Geometry check sheet. Reference: the model listing, model coordinates, mm. Give positions to 0.01 mm unless a question says otherwise; leave off trailing zeros. Loops run counter-clockwise (first coordinate to the right, second up) from the corner with the lowest first, then second, coordinate; pieces in that order, holes last. Notation, with made-up numbers: (-29, 39.25) -> (-2, 39.25) arc R10 ccw to (-2, 45.25) -> close; hole circle Ø11 at (89, -2.5). An arc over 180 degrees is marked (long way). One line per question, with ' | ' between items.
from build123d import *

# Parameters (mm, degrees)
F0_R     = 10
F0_R_2   = 1.75
F1_DEPTH = 3
F2_SIZE  = 0.5
F3_SIZE2 = 0.6
F3_SIZE  = 0.4


with BuildPart() as f1:
    # F0 (on Right) → F1 (new body)
    with BuildSketch(Plane.YZ):
        Circle(F0_R)
        with Locations((0, -6.35)):
            Circle(F0_R_2, mode=Mode.SUBTRACT)
        with Locations((-6.35, 0)):
            Circle(F0_R_2, mode=Mode.SUBTRACT)
        with Locations((6.35, 0)):
            Circle(F0_R_2, mode=Mode.SUBTRACT)
        with Locations((0, 6.35)):
            Circle(F0_R_2, mode=Mode.SUBTRACT)
    extrude(amount=F1_DEPTH)

    # F2
    f2_edges = [f1.edges().sort_by_distance(p)[0] for p in [
        (3, -8.1, 0),
        (3, -1.75, 6.35),
        (3, 4.6, 0),
        (3, -1.75, -6.35),
    ]]
    chamfer(f2_edges, length=F2_SIZE)

    # F3
    f3_edges = [f1.edges().sort_by_distance(p)[0] for p in [
        (3, -10, 0),
        (0, -10, 0),
    ]]
    chamfer(f3_edges, length=F3_SIZE, length2=F3_SIZE2)


solid = f1.part
Item 1: Scan lines: probe 1 along Z at (x, y) = (2.05, 0); probe 2 along Y at (x, z) = (1.45, 0.5); probe 3 along Z at (x, y) = (2.7, -6). Record each from-to range of solid material in increasing order.
Result:
probe 1: -10 to -8.1, -4.6 to 4.6, 8.1 to 10 | probe 2: -9.99 to -8.03, -4.67 to 4.67, 8.03 to 9.99 | probe 3: -7.75 to -1.92, 1.92 to 7.75
Item 2: Release check for a two-part mould opening along Z. For faces 1 (the face through (1.232, 0.941, -4.874)), 2 (the face through (0, 0, 0)), 3 (the face through (1.49, -2.17, -9.76)) record: pulls with the +Z half, pulls with the -Z half, needs draft (parallel to the pull), parting line crosses it, or undercut.
Result:
face 1: undercut | face 2: needs draft | face 3: parting line crosses it
Item 3: Depth check by flat-ended pin: pin 1 Ø1 at (x, z) = (1, 7.5) entering from -Y; pin 2 Ø3 at (y, z) = (0, -6.35) entering from -X. Enter the tip coordinate at first touch or a pass-through.
Result:
pin 1: y = -7.14 | pin 2: through
Item 4: Sectioned sample at A-A (z = 0). Record the cut outline in (x, y), plus the area to 3 significant figures.
Result:
outline: (0, -9.6) -> (0.6, -10) -> (2.4, -10) -> (3, -9.6) -> (3, -8.6) -> (2.5, -8.1) -> (0, -8.1) -> close; (0, -4.6) -> (2.5, -4.6) -> (3, -4.1) -> (3, 4.1) -> (2.5, 4.6) -> (0, 4.6) -> close; (0, 8.1) -> (2.5, 8.1) -> (3, 8.6) -> (3, 9.6) -> (2.4, 10) -> (0.6, 10) -> (0, 9.6) -> close | area: 38.0 mm2
